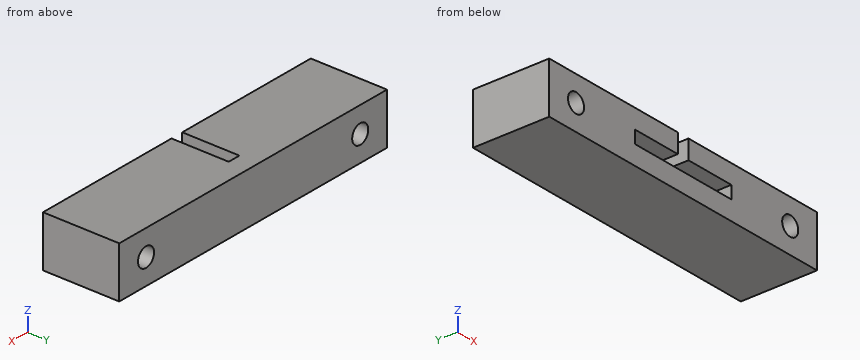
from build123d import *

# Parameters (mm, degrees)
F0_W     = 50
F0_H     = 12
F1_DEPTH = 8
F2_R     = 1.5
F3_DEPTH = 12
F4_DEPTH = 9


with BuildPart() as f1:
    # F0 (on Top) → F1 (new body)
    with BuildSketch(Plane.XY):
        with Locations((25, 6)):
            Rectangle(F0_W, F0_H)
    extrude(amount=F1_DEPTH)

    # F2 (on face) → F3 (cut)
    with BuildSketch(Plane.XZ):
        with Locations((5, 4)):
            Circle(F2_R)
        with Locations((45, 4)):
            Circle(F2_R)
    extrude(amount=-F3_DEPTH, mode=Mode.SUBTRACT)

    # F2 (on face) → F4 (cut)
    with BuildSketch(Plane.XZ):
        Polygon((26, 8), (24, 8), (24, 5), (16, 5), (16, 3), (34, 3), (34, 5), (26, 5), align=None)
    extrude(amount=-F4_DEPTH, mode=Mode.SUBTRACT)


solid = f1.part
Could you check a few things on this model? Use its own coordinates, in mm. Coordinates: 2 decimals unless noted, no trailing zeros. Loops run counter-clockwise (first coordinate to the right, second up) from the corner with the lowest first, then second, coordinate; pieces in that order, holes last.
1. I need wall thicknesses on L1, parallel to X at y = 10.25, z = 3.25; L2, parallel to X at y = 3.25, z = 3.25; L3, parallel to Z at x = 23.5, y = 7.75. Which ranges of each line are inside material? Lowest first, please.
2. Imagine slicing it at D-D (z = 7). Please give me the cut outline in (x, y).
3. Imagine slicing it at B-B (y = 11). Please give me the cut outline in (x, z).
4. Imagine slicing it at C-C (z = 4). Please give me the cut outline in (x, y), and give its area (3 significant figures).
5. For P1, Ø2.5, axis at x = 45, z = 4, coming from the +Y side, with a flat end and sliding along its axis, tell me the tip position at first contact or that it passes through.
6. Imagine slicing it at A-A (x = 45). Please give me the cut outline in (y, z).
Computed values:
1. L1: x = 0 to 3.7, 6.3 to 43.7, 46.3 to 50
1. L2: x = 0 to 3.7, 6.3 to 16, 34 to 43.7, 46.3 to 50
1. L3: z = 0 to 3, 5 to 8
2. outline: (0, 0) - (24, 0) - (24, 9) - (26, 9) - (26, 0) - (50, 0) - (50, 12) - (0, 12) - close
3. outline: (0, 0) - (50, 0) - (50, 8) - (0, 8) - close; hole circle Ø3 at (5, 4); hole circle Ø3 at (45, 4)
4. outline: (0, 0) - (3.5, 0) - (3.5, 12) - (0, 12) - close; (6.5, 0) - (16, 0) - (16, 9) - (34, 9) - (34, 0) - (43.5, 0) - (43.5, 12) - (6.5, 12) - close; (46.5, 0) - (50, 0) - (50, 12) - (46.5, 12) - close
4. area: 366 mm2
5. P1: passes through
6. outline: (0, 0) - (12, 0) - (12, 2.5) - (0, 2.5) - close; (0, 5.5) - (12, 5.5) - (12, 8) - (0, 8) - close
